Autodesk Inventor part; units mm, degrees
ref_plane "YZ Plane" through (0, 0, 0) normal (1, 0, 0) x (0, 1, 0)
ref_plane "XZ Plane" through (0, 0, 0) normal (0, 1, 0) x (-1, 0, 0)
ref_plane "XY Plane" through (0, 0, 0) normal (0, 0, 1) x (1, 0, 0)
sketch "Sketch1" plane through (0, 0, 0) normal (0, 0, 1) x (1, 0, 0)
  circle A0 centre (4.9, 17.1) radius 0.455
  circle A1 centre (4.9, 17.1) radius 0.7
  line L0 (6.3, 15.875) -> (6.3, 17.1)
  line L1 (0, 31) -> (7, 31)
  line L2 (7, 31) -> (7, 29.75)
  line L3 (7, 29.75) -> (1.75, 29.75)
  line L4 (0, 0) -> (9.5856, 0)
  line L5 (0, 31) -> (0, 17.1)
  line L6 (0, 17.1) -> (1.75, 16.75)
  line L7 (1.75, 16.75) -> (4.9, 15)
  line L8 (4.9, 15) -> (6.3, 15.875)
  line L9 (4.9, 15) -> (0, 15) construction
  line L10 (0, 31.2) -> (0, -5.2)
  line L11 (-1.9171, 0) -> (11.5027, 0)
  line L12 (4.2, 17.1) -> (1.75, 17.59)
  line L13 (1.75, 17.59) -> (1.75, 29.75)
  line L14 (6.3, 17.1) -> (5.6, 17.1)
  dimension "d0" = 62
  dimension "d1" = 31.75
  dimension "d2" = 1.25
  dimension "d3" = 0.91
  dimension "d4" = 1.4
  dimension "d5" = 30
  dimension "d6" = 33.5
  dimension "d7" = 34.2
  dimension "d8" = 4.9
  dimension "d9" = 6.3
  dimension "d10" = 7
  dimension "d12" = 1.75
revolve "Body" add sketch "Sketch1" angle 360 about axis through (0, 0, 0) along (1, 0, 0) contours L14 L0 L8 L7 L6 L5 L1 L2 L3 L13 L12 A1
revolve "Spring1" add sketch "Sketch1" angle 360 about axis through (0, 0, 0) along (1, 0, 0) contours A0 | A1
fillet "Fillet1" radius 0.4 3 edges at (7, -31, 0) (1.75, -29.75, 0) (0, -31, 0)
equation "\"d0\" = SD2"
equation "\"d1\" = ABDM"
equation "\"d3\" = SPDI"
equation "\"d4\" = SPDA"
equation "\"d5\" = NND"
equation "\"d6\" = TKDM"
equation "\"d7\" = HLDM"
equation "\"d8\" = SPDST"
equation "\"d9\" = SDI"
equation "\"d10\" = SWDT"
equation "\"d12\" = SD"
equation "\"d11\" = RR"
equation "\"SD2\" = 62"
equation "\"SWDT\" = 7"
equation "\"RR\" = 0.4"
equation "\"SD\" = 1.75"
equation "\"NND\" = 30"
equation "\"SPDA\" = 1.4"
equation "\"SPDI\" = 0.91"
equation "\"TKDM\" = 33.5"
equation "\"HLDM\" = 34.2"
equation "\"ABDM\" = 31.75"
equation "\"SDI\" = 6.3"
equation "\"SPDST\" = 4.9"
equation "\"LAB\" = 0.35"
properties part number "PWTR-0069" material "Rubber"
Verification items for the finished model (mm, model axes). A direction names the side the tool comes from. Coordinates: 2 decimals unless noted, no trailing zeros. Return JSON: item names as keys, results as strings.
1) Release check for a two-part mould opening along Z. For faces 1 (the flat face through (0, 13, -13)), 2 (the cylindrical face through (3.543, -4.036, 30.736)), 3 (the conical face through (4.047, 16.34, -5.146)) record: +Z half, -Z half, draft (parallel to the pull), parting line (faces both ways), or undercut.
Answer list:
{"face 1": "draft", "face 2": "parting line", "face 3": "undercut"}
2) Gauge pin test, flat ends, axial feed: pin 1 (1.5 mm diameter, centred on x = 4, y = -13, fed in from -Z); pin 2 (1.5 mm diameter, centred on x = 5, z = -15.5, fed in from -Y); pin 3 (17.5 mm diameter, centred on y = -7, z = 7, fed in from +X). Record the tip position at first contact, or that the pin passes through.
Answer list:
{"pin 1": "z = -28.48", "pin 2": "y = -27.27", "pin 3": "x = 6.3"}
3) Thickness scan on L1, parallel to Z at x = 4.7, y = 0; L2, parallel to Y at x = 4, z = -3; L3, parallel to Y at x = 2.25, z = 10.5. Record the ranges inside material, lowest first. Write a range as [from, to].
Answer list:
{"L1": "[-31, -29.75], [-17.77, -15.11], [15.11, 17.77], [29.75, 31]", "L2": "[-30.85, -29.6], [-16.88, -15.21], [15.21, 16.88], [29.6, 30.85]", "L3": "[-29.17, -27.84], [-13.99, -12.69], [12.69, 13.99], [27.84, 29.17]"}
4) Access from +Z, -Z, +X, -X, +Y, -Y to the whole of each face (thin tool, end or side, straight path). Record for faces 4 (the conical face through (4.7, -3.28, 14.75)), 5 (the flat face through (6.3, 10, -13)).
Answer list:
{"face 4": "-X", "face 5": "+X"}
